Can you work these out from the model? Positions are in its coordinate system, mm. A direction names the side the tool comes from. Coordinates: 2 decimals unless noted, no trailing zeros. Order: outer loops, then holes, each group sorted by start corner. A loop starts at its lowest first (then second) coordinate and runs counter-clockwise, first axis right, second up. Notation, with made-up numbers: (14.25, -5) -> (40.25, -5) arc R16 cw to (40.25, 1) -> close; hole circle Ø10 at (17.25, -18). An arc over 180 degrees is marked (long way). Answer in a Markdown table with one row per item.
```python
from build123d import *

# Parameters (mm, degrees)
SKETCH1_W               = 130
SKETCH1_H               = 210
BOSS_EXTRUDE1_DEPTH     = 3
FILLET1_R               = 20
FILLET2_R               = 20
SKETCH2_W               = 25
SKETCH2_H               = 10
BOSS_EXTRUDE2_DEPTH     = 10
MIRROR2_COPY_1_SKETCH_W = 25
MIRROR2_COPY_1_SKETCH_H = 10
MIRROR2_COPY_1_DEPTH    = 10
SKETCH3_W               = 67
SKETCH3_H               = 60
SKETCH3_W_2             = 61
SKETCH3_H_2             = 54
BOSS_EXTRUDE3_DEPTH     = 3
CROQUIS1_R              = 1.6
CORTAR_EXTRUIR1_DEPTH   = 10
CROQUIS2_R              = 1.75
CORTAR_EXTRUIR2_DEPTH   = 10


with BuildPart() as part:
    # Sketch1 → Boss-Extrude1 (new body)
    with BuildSketch(Plane.XY):
        Rectangle(SKETCH1_W, SKETCH1_H)
    extrude(amount=BOSS_EXTRUDE1_DEPTH)

    # Fillet1
    fillet1_edges = [part.edges().sort_by_distance(p)[0] for p in [
        (-65, 105, 1.5),
    ]]
    fillet(fillet1_edges, radius=FILLET1_R)

    # Fillet2
    fillet2_edges = [part.edges().sort_by_distance(p)[0] for p in [
        (65, 105, 1.5),
    ]]
    fillet(fillet2_edges, radius=FILLET2_R)

    # Sketch2 → Boss-Extrude2 (add)
    with BuildSketch(Plane.XY.offset(3)):
        with Locations((52.3, 53.9)):
            Rectangle(SKETCH2_W, SKETCH2_H)
        with Locations((52.3, 76.1)):
            Rectangle(SKETCH2_W, SKETCH2_H)
    boss_extrude2 = extrude(amount=BOSS_EXTRUDE2_DEPTH)

    # Mirror1: Boss-Extrude2 across plane
    add(boss_extrude2.mirror(Plane.ZX))

    # Mirror2: Boss-Extrude2 across plane
    add(boss_extrude2.mirror(Plane(origin=(0, 0, 0), x_dir=(0, 0, 1), z_dir=(1, 0, 0))))

    # Mirror2 copy 1 sketch → Mirror2 copy 1 (add)
    with BuildSketch(Plane(origin=(0, 0, 3), x_dir=(-1, 0, 0), z_dir=(0, 0, 1))):
        with Locations((52.3, 53.9)):
            Rectangle(MIRROR2_COPY_1_SKETCH_W, MIRROR2_COPY_1_SKETCH_H)
        with Locations((52.3, 76.1)):
            Rectangle(MIRROR2_COPY_1_SKETCH_W, MIRROR2_COPY_1_SKETCH_H)
    extrude(amount=MIRROR2_COPY_1_DEPTH)

    # Sketch3 → Boss-Extrude3 (add)
    with BuildSketch(Plane.XY.offset(3)):
        with Locations((0, 28.5)):
            Rectangle(SKETCH3_W, SKETCH3_H)
        with Locations((0, 28.5)):
            Rectangle(SKETCH3_W_2, SKETCH3_H_2, mode=Mode.SUBTRACT)
    boss_extrude3 = extrude(amount=BOSS_EXTRUDE3_DEPTH)

    # Mirror3: Boss-Extrude3 across plane
    add(boss_extrude3.mirror(Plane.ZX))

    # Croquis1 → Cortar-Extruir1 (cut)
    with BuildSketch(Plane.XY.offset(3)):
        with Locations((-15, 85)):
            Circle(CROQUIS1_R)
        with Locations((15, 69.5)):
            Circle(CROQUIS1_R)
        with Locations((-15.5, -70)):
            Circle(CROQUIS1_R)
        with Locations((15.5, -85)):
            Circle(CROQUIS1_R)
    extrude(amount=-CORTAR_EXTRUIR1_DEPTH, mode=Mode.SUBTRACT)

    # Croquis2 → Cortar-Extruir2 (cut)
    with BuildSketch(Plane.XY.offset(3)):
        with Locations((-61, -101)):
            Circle(CROQUIS2_R)
        with Locations((61, -101)):
            Circle(CROQUIS2_R)
        with Locations((56, 96)):
            Circle(CROQUIS2_R)
        with Locations((-56, 96)):
            Circle(CROQUIS2_R)
    extrude(amount=-CORTAR_EXTRUIR2_DEPTH, mode=Mode.SUBTRACT)


solid = part.part
```
(1) Suppose I cut it at C-C (x = 9). Please give me the cut outline in (y, z).
Response values:
| item | result |
|---|---|
| outline | (-105, 0) -> (105, 0) -> (105, 3) -> (58.5, 3) -> (58.5, 6) -> (55.5, 6) -> (55.5, 3) -> (1.5, 3) -> (1.5, 6) -> (-1.5, 6) -> (-1.5, 3) -> (-55.5, 3) -> (-55.5, 6) -> (-58.5, 6) -> (-58.5, 3) -> (-105, 3) -> close |
(2) On a 3-axis mill with a long thin cutter (end or side, diameter ignored), from which of +Z, -Z, +X, -X, +Y, -Y can I reach the whole of each face in a straight line? I mean faces 5 (the flat face through (52, -81.1, 8)), 6 (the flat face through (-52, 48.9, 8)), 7 (the flat face through (0, 0, 6)), 8 (the flat face through (64.8, 76, 8)). Say none if no direction works.
Response values:
| item | result |
|---|---|
| face 5 | +Z, +X, -X, -Y |
| face 6 | +Z, -X |
| face 7 | +Z, +Y, -Y |
| face 8 | +Z, +X, +Y, -Y |
(3) I need wall thicknesses on line 1 (X direction, y = -101, z = 1.1); line 2 (Y direction, x = -15, z = 1.45); line 3 (Y direction, x = 15.5, z = 1). Which ranges of each line are inside material? Lowest first, please. Write a range as [from, to].
Response values:
| item | result |
|---|---|
| line 1 | [-65, -62.75], [-59.25, 59.25], [62.75, 65] |
| line 2 | [-105, -71.52], [-68.48, 83.4], [86.6, 105] |
| line 3 | [-105, -86.6], [-83.4, 67.98], [71.02, 105] |
(4) Will these pins go through, and if not, where does the flat tip stop? pin 1 Ø12 at (x, y) = (1, -5) entering from +Z; pin 2 Ø4 at (x, y) = (15, 69.5) entering from -Z; pin 3 Ø4 at (x, y) = (-27, -76.5) entering from +Z; pin 4 Ø3 at (x, z) = (56, 9.5) entering from +Y.
Response values:
| item | result |
|---|---|
| pin 1 | z = 6 |
| pin 2 | z = 0 |
| pin 3 | z = 3 |
| pin 4 | y = 81.1 |
(5) Suppose I cut it at D-D (y = 51.5). Please give me the cut outline in (x, z).
Response values:
| item | result |
|---|---|
| outline | (-65, 0) -> (65, 0) -> (65, 3) -> (64.8, 3) -> (64.8, 13) -> (39.8, 13) -> (39.8, 3) -> (33.5, 3) -> (33.5, 6) -> (30.5, 6) -> (30.5, 3) -> (-30.5, 3) -> (-30.5, 6) -> (-33.5, 6) -> (-33.5, 3) -> (-39.8, 3) -> (-39.8, 13) -> (-64.8, 13) -> (-64.8, 3) -> (-65, 3) -> close |
(6) Suppose I cut it at B-B (y = -39). Please give me the cut outline in (x, z).
Response values:
| item | result |
|---|---|
| outline | (-65, 0) -> (65, 0) -> (65, 3) -> (33.5, 3) -> (33.5, 6) -> (30.5, 6) -> (30.5, 3) -> (-30.5, 3) -> (-30.5, 6) -> (-33.5, 6) -> (-33.5, 3) -> (-65, 3) -> close |
(7) Suppose I cut it at A-A (z = 10.75). Count the separate pieces of the cut face and the enclosed holes in it, and give its area (3 significant figures).
Response values:
| item | result |
|---|---|
| separate pieces | 8 |
| enclosed holes | 0 |
| area | 2,000 mm2 |
(8) We'd pull the mould along Y, two halves only. Please class faces 1 (the flat face through (0, 29, 3)), 2 (the flat face through (52, 48.9, 8)), 3 (the cylindrical face through (58.986, 99.297, 1.521)), 4 (the flat face through (39.8, -54, 8)): +Y half, -Y half, draft (parallel to the pull), parting line (faces both ways), or undercut.
Response values:
| item | result |
|---|---|
| face 1 | undercut |
| face 2 | undercut |
| face 3 | +Y half |
| face 4 | draft |
